Geometry check sheet. Reference: the model listing, model coordinates, mm. A direction names the side the tool comes from. Coordinates: 2 decimals unless noted, no trailing zeros. Order: outer loops, then holes, each group sorted by start corner. A loop starts at its lowest first (then second) coordinate and runs counter-clockwise, first axis right, second up. Notation, with made-up numbers: (35.5, 62.5) - (46.5, 62.5) arc R18 cw to (46.5, 76.5) - close; hole circle Ø6 at (8.25, -27). An arc over 180 degrees is marked (long way). Return JSON: item names as keys, results as strings. Group by question number.
Item 1: Section check B-B on x = 0. Enter the section's corners in (y, z), then the cut area to 3 significant figures.
Item 2: Tool access check on faces 1 (the flat face through (0, 5, -6.75)), 2 (the flat face through (-5.87, 5.22, 3.33)), 3 (the cylindrical face through (-5, 1.5, 8.6)), 4 (the cylindrical face through (-3.81, 5.28, -6.62)), 5 (the flat face through (0, 1, 8.75)). Record the directions out of +Z, -Z, +X, -X, +Y, -Y that give a thin tool (end or side, any length) a straight path to the whole face; none if there is none.
Item 3: Section check A-A on y = 4. Enter the section's corners in (x, z).
Item 4: Scan lines: probe 1 along Z at (x, y) = (0, 5.45); probe 2 along Z at (x, y) = (0, 2.4); probe 3 along Y at (x, z) = (-7.5, -1.25). Record each from-to range of solid material in increasing order.
Item 5: Gauge pin test, flat ends, axial feed: pin 1 (1 mm diameter, centred on x = 3.5, y = 4.5, fed in from +Z); pin 2 (3.5 mm diameter, centred on x = 1, y = 5, fed in from -Z); pin 3 (2 mm diameter, centred on x = 5, y = 5.5, fed in from -Z); pin 4 (10 mm diameter, centred on x = -0.5, z = 1, fed in from -Y). Record the tip position at first contact, or that the pin passes through.
from build123d import *

# Parameters (mm, degrees)
BOSS_EXTRUDE1_DEPTH                      = 3
BOSS_EXTRUDE2_DEPTH                      = 5
CBORE_FOR_M4_PAN_HEAD_SCREW1_D           = 4.5
CBORE_FOR_M4_PAN_HEAD_SCREW1_CBORE_D     = 9
CBORE_FOR_M4_PAN_HEAD_SCREW1_CBORE_DEPTH = 3.1
FILLET1_R                                = 1
FILLET2_R                                = 1
FILLET5_R                                = 0.5
FILLET6_R                                = 0.5
FILLET7_R                                = 0.5


with BuildPart() as part:
    # Sketch1 → Boss-Extrude1 (new body)
    with BuildSketch(Plane(origin=(0, 0, 0), x_dir=(1, 0, 0), z_dir=(0, 1, 0))):
        Polygon((10.103629711, 0), (5.051814855, 8.75), (-5.051814855, 8.75), (-10.103629711, 0), (-5.051814855, -8.75), (5.051814855, -8.75), align=None)
    extrude(amount=BOSS_EXTRUDE1_DEPTH)

    # Sketch2 → Boss-Extrude2 (add)
    with BuildSketch(Plane(origin=(0, 3, 0), x_dir=(1, 0, 0), z_dir=(0, 1, 0))):
        Polygon((3.897114317, -6.75), (7.794228634, 0), (3.897114317, 6.75), (-3.897114317, 6.75), (-7.794228634, 0), (-3.897114317, -6.75), align=None)
    extrude(amount=BOSS_EXTRUDE2_DEPTH)

    # CBORE for M4 Pan Head Screw1 (through all)
    with Locations(Plane.XZ):
        with Locations((0, 0)):
            CounterBoreHole(CBORE_FOR_M4_PAN_HEAD_SCREW1_D / 2, CBORE_FOR_M4_PAN_HEAD_SCREW1_CBORE_D / 2, CBORE_FOR_M4_PAN_HEAD_SCREW1_CBORE_DEPTH)

    # Fillet1
    fillet1_edges = [part.edges().sort_by_distance(p)[0] for p in [
        (-3.897114317, 5.5, 6.75),
        (3.897114317, 5.5, 6.75),
        (7.794228634, 5.5, 0),
        (3.897114317, 5.5, -6.75),
        (-3.897114317, 5.5, -6.75),
        (-7.794228634, 5.5, 0),
    ]]
    fillet(fillet1_edges, radius=FILLET1_R)

    # Fillet2
    fillet2_edges = [part.edges().sort_by_distance(p)[0] for p in [
        (5.051814855, 1.5, 8.75),
        (-5.051814855, 1.5, 8.75),
        (-10.103629711, 1.5, 0),
        (-5.051814855, 1.5, -8.75),
        (5.051814855, 1.5, -8.75),
        (10.103629711, 1.5, 0),
    ]]
    fillet(fillet2_edges, radius=FILLET2_R)

    # Fillet5
    fillet5_edges = [part.edges().sort_by_distance(p)[0] for p in [
        (5.845671476, 8, -3.375),
        (5.845671476, 8, 3.375),
        (0, 8, 6.75),
        (0, 8, -6.75),
        (-5.845671476, 8, -3.375),
        (-5.845671476, 8, 3.375),
        (3.819764048, 8, -6.616025404),
        (-3.819764048, 8, -6.616025404),
        (-7.639528096, 8, 0),
        (-3.819764048, 8, 6.616025404),
        (3.819764048, 8, 6.616025404),
        (7.639528096, 8, 0),
    ]]
    fillet(fillet5_edges, radius=FILLET5_R)

    # Fillet6
    fillet6_edges = [part.edges().sort_by_distance(p)[0] for p in [
        (-4.5, 0, 0),
        (-7.577722283, 0, 4.375),
        (7.577722283, 0, 4.375),
        (0, 0, 8.75),
        (-7.577722283, 0, -4.375),
        (0, 0, -8.75),
        (7.577722283, 0, -4.375),
        (-4.974464586, 0, 8.616025404),
        (4.974464586, 0, 8.616025404),
        (9.948929172, 0, 0),
        (4.974464586, 0, -8.616025404),
        (-4.974464586, 0, -8.616025404),
        (-9.948929172, 0, 0),
    ]]
    fillet(fillet6_edges, radius=FILLET6_R)

    # Fillet7
    fillet7_edges = [part.edges().sort_by_distance(p)[0] for p in [
        (-4.974464586, 3, 8.616025404),
        (4.974464586, 3, 8.616025404),
        (9.948929172, 3, 0),
        (4.974464586, 3, -8.616025404),
        (-4.974464586, 3, -8.616025404),
        (-9.948929172, 3, 0),
        (-7.577722283, 3, 4.375),
        (-7.577722283, 3, -4.375),
        (7.577722283, 3, 4.375),
        (7.577722283, 3, -4.375),
        (0, 3, -8.75),
        (0, 3, 8.75),
    ]]
    fillet(fillet7_edges, radius=FILLET7_R)


solid = part.part
Computed:
{
 "1": {"outline": "(0, -8.25) arc R0.5 ccw to (0.5, -8.75) - (2.5, -8.75) arc R0.5 ccw to (3, -8.25) - (3, -6.75) - (7.5, -6.75) arc R0.5 ccw to (8, -6.25) - (8, -2.25) - (3.1, -2.25) - (3.1, -4.5) - (0.5, -4.5) arc R0.5 ccw to (0, -5) - close; (0, 5) arc R0.5 ccw to (0.5, 4.5) - (3.1, 4.5) - (3.1, 2.25) - (8, 2.25) - (8, 6.25) arc R0.5 ccw to (7.5, 6.75) - (3, 6.75) - (3, 8.25) arc R0.5 ccw to (2.5, 8.75) - (0.5, 8.75) arc R0.5 ccw to (0, 8.25) - close", "area": "69.6 mm²"},
 "2": {"face 1": "-Z, +X, -X, +Y", "face 2": "+Z, -X, +Y", "face 3": "+Z, -X, +Y, -Y", "face 4": "-Z, -X, +Y", "face 5": "+Z, +X, -X, +Y, -Y"},
 "3": {"outline": "(-7.51, -0.5) - (-4.19, -6.25) arc R1 ccw to (-3.32, -6.75) - (3.32, -6.75) arc R1 ccw to (4.19, -6.25) - (7.51, -0.5) arc R1 ccw to (7.51, 0.5) - (4.19, 6.25) arc R1 ccw to (3.32, 6.75) - (-3.32, 6.75) arc R1 ccw to (-4.19, 6.25) - (-7.51, 0.5) arc R1 ccw to start; hole circle Ø4.5 at (0, 0)"},
 "4": {"probe 1": "z = -6.75 to -2.25, 2.25 to 6.75", "probe 2": "z = -8.75 to -4.5, 4.5 to 8.75", "probe 3": "y = 0 to 3"},
 "5": {"pin 1": "stops at z = 6.75", "pin 2": "stops at z = -6.75", "pin 3": "stops at z = -6.48", "pin 4": "stops at y = 0"}
}
